Design review of the part built by this model. Coordinates are the model's own, in mm. Face numbers are marked on the shaded views. Give positions to 0.01 mm unless a question says otherwise; leave off trailing zeros. Order: outer loops, then holes, each group sorted by start corner. A loop starts at its lowest first (then second) coordinate and runs counter-clockwise, first axis right, second up. Notation, with made-up numbers: (79.25, 29.5) -> (114.25, 29.5) arc R10 ccw to (114.25, 46.5) -> close; hole circle Ø9 at (44.5, -9). An arc over 180 degrees is marked (long way). One line per item, written item: value. Start each with the question number.
1) The part is to be moulded in two halves that separate along Y. For the marked faces 1, 2, 3 and 4, say which applies: released by +Y, released by -Y, zero draft, split by the parting line, or undercut.
2) For pin 1 (3 mm diameter, centred on x = -18.5, y = -44, fed in from +Z); pin 2 (3.5 mm diameter, centred on y = 56, z = 9.5, fed in from +X); pin 3 (2 mm diameter, centred on x = 1, y = 43.5, fed in from -Z), all flat-tipped, find the tip position at first contact; note any pin that passes through.
3) Wall thickness on line 1 along Y through (x, z) = (23.5, 4.25); line 2 along Y through (x, z) = (24.5, 7.25); line 3 along X through (y, z) = (-49, 11.25): over which ranges is each line inside the solid? List them lowest first. Write a range as from..to.
4) Consider section D-D (x = -26). State the section outline as (y, z) points, plus the area to 3 significant figures.
5) Consider section C-C (x = -14). State the section outline as (y, z) points, plus the area to 3 significant figures.
6) Consider section B-B (z = 2.5). State the section outline as (x, y) points.
7) Consider section A-A (y = 27). State the section outline as (x, z) points, plus the area to 3 significant figures.
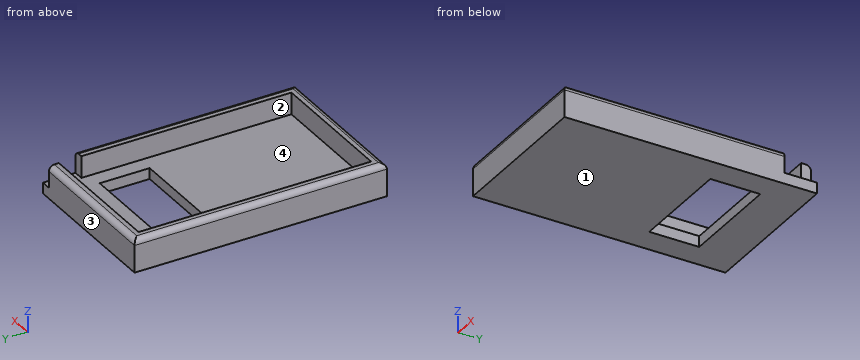
from build123d import *

# Parameters (mm, degrees)
F0_W     = 47.5
F0_H     = 23
F1_DEPTH = 5
F2_DEPTH = 15
F3_R     = 2.5


with BuildPart() as f1:
    # F0 (on Top) → F1 (new body)
    with BuildSketch(Plane.XY):
        Polygon((35.5799995661, 43.7052872479), (35.5799995661, 58.0799995661), (31, 58.0799995661), (31, 53.5), (31, 43.15), (35.5799995661, 43.15), align=None)
        Polygon((31, 53.5), (31, 58.0799995661), (-35.5799995661, 58.0799995661), (-35.5799995661, -58.0799995661), (35.5799995661, -58.0799995661), (35.5799995661, 43.15), (31, 43.15), (31, -53.5), (-31, -53.5), (-31, 53.5), align=None)
        Polygon((31, 43.15), (31, 53.5), (-31, 53.5), (-31, -53.5), (31, -53.5), align=None)
        with Locations((0, 27.5)):
            Rectangle(F0_W, F0_H, mode=Mode.SUBTRACT)
    extrude(amount=F1_DEPTH)

    # F0 (on Top) → F2 (join)
    with BuildSketch(Plane.XY):
        Polygon((31, 53.5), (31, 58.0799995661), (-35.5799995661, 58.0799995661), (-35.5799995661, -58.0799995661), (35.5799995661, -58.0799995661), (35.5799995661, 43.15), (31, 43.15), (31, -53.5), (-31, -53.5), (-31, 53.5), align=None)
    extrude(amount=F2_DEPTH)

    # F3
    f3_edges = [f1.edges().sort_by_distance(p)[0] for p in [
        (-35.58, 0, 15),
        (-2.29, 58.08, 15),
        (0, -58.08, 15),
        (35.58, -7.465, 15),
    ]]
    fillet(f3_edges, radius=F3_R)


solid = f1.part
Checked values:
1. face 1: zero draft
1. face 2: undercut
1. face 3: released by +Y
1. face 4: undercut
2. pin 1: stops at z = 5
2. pin 2: stops at x = 31
2. pin 3: stops at z = 0
3. line 1: y = -58.08..16, 39..58.08
3. line 2: y = -58.08..-53.5, 53.5..58.08
3. line 3: x = -35.58..-31, 31..35.58
4. outline: (-58.08, 0) -> (58.08, 0) -> (58.08, 12.5) arc R2.5 ccw to (55.58, 15) -> (53.5, 15) -> (53.5, 5) -> (-53.5, 5) -> (-53.5, 15) -> (-55.58, 15) arc R2.5 ccw to (-58.08, 12.5) -> close
4. area: 670 mm^2
5. outline: (-58.08, 0) -> (16, 0) -> (16, 5) -> (-53.5, 5) -> (-53.5, 15) -> (-55.58, 15) arc R2.5 ccw to (-58.08, 12.5) -> close; (39, 0) -> (58.08, 0) -> (58.08, 12.5) arc R2.5 ccw to (55.58, 15) -> (53.5, 15) -> (53.5, 5) -> (39, 5) -> close
5. area: 555 mm^2
6. outline: (-35.58, -58.08) -> (35.58, -58.08) -> (35.58, 58.08) -> (-35.58, 58.08) -> close; hole (-23.75, 16) -> (23.75, 16) -> (23.75, 39) -> (-23.75, 39) -> close
7. outline: (-35.58, 0) -> (-23.75, 0) -> (-23.75, 5) -> (-31, 5) -> (-31, 15) -> (-33.08, 15) arc R2.5 ccw to (-35.58, 12.5) -> close; (23.75, 0) -> (35.58, 0) -> (35.58, 12.5) arc R2.5 ccw to (33.08, 15) -> (31, 15) -> (31, 5) -> (23.75, 5) -> close
7. area: 207 mm^2
